Geometry: final body of the model. Coordinates: model frame, mm. Face numbers are marked on the shaded views. Round coordinates to 2 decimals unless told otherwise and drop trailing zeros. Order: outer loops, then holes, each group sorted by start corner. A loop starts at its lowest first (then second) coordinate and runs counter-clockwise, first axis right, second up. Notation, with made-up numbers: M 80,54.25 L 126,54.25 A19 cw 126,83.25 Z; hole C 89,18.25 d9. An arc over 180 degrees is marked long. Return JSON: item names as keys, results as strings. Group by question number.
Q1. Cut plane B-B on y = 15. Output: boundary loops of the cut face in (x, z).
Q2. Cut plane A-A on y = 10. Output: boundary loops of the cut face in (x, z), and give its area (3 significant figures).
Q3. Mould query, pull axis Y, two halves, no side actions, for the marked faces 1, 2 and 3. Classes: released by +Y, released by -Y, zero draft, split by the parting line, or undercut.
Q4. Ray query, probe 1 along X at (y, z) = (10, 2.15); probe 2 along X at (y, z) = (16, 2); probe 3 along Y at (x, z) = (14, 17.5) (3 decimals). Return the intervals inside material, ascending.
Q5. Contact query for flat-ended pins moving along their axis: pin 1 (2.5 mm diameter, centred on x = 15, y = 10, fed in from +Z); pin 2 (1.5 mm diameter, centred on x = 6, y = 11, fed in from -Z); pin 3 (10 mm diameter, centred on x = 8, y = 10.5, fed in from +Z); pin 4 (5.5 mm diameter, centred on y = 6.5, z = 1.5, fed in from -X). Output: stop coordinate, or through.
```python
from build123d import *

# Parameters (mm, degrees)
ESQUISSE1_W                                       = 10
ESQUISSE1_H                                       = 20
ESQUISSE1_W_2                                     = 20
BOSS_EXTRU_3_DEPTH                                = 5
BOSS_EXTRU_5_DEPTH                                = 2
ESQUISSE15_W                                      = 8
ESQUISSE15_H                                      = 17.913431031
BOSS_EXTRU_6_DEPTH                                = 0.1
ESQUISSE16_W                                      = 1
ESQUISSE16_H                                      = 17.913431031
BOSS_EXTRU_7_DEPTH                                = 1
BOSS_EXTRU_11_DEPTH                               = 2
ESQUISSE32_W                                      = 8
ESQUISSE32_H                                      = 17.913431031
BOSS_EXTRU_14_DEPTH                               = 0.125
ESQUISSE42_R                                      = 1.279103286
BOSS_EXTRU_18_DEPTH                               = 7
ESQUISSE56_R                                      = 1.3
BOSS_EXTRU_20_DEPTH                               = 7
CONG_4_R                                          = 1
ESQUISSE33_W                                      = 1
ESQUISSE33_H                                      = 17.913431031
BOSS_EXTRU_15_DEPTH                               = 1
ESQUISSE35_R                                      = 2.128247198
ENL_V_MAT_EXTRU_1_DEPTH                           = 5
ESQUISSE37_W                                      = 26
ESQUISSE37_H                                      = 16
ENL_V_MAT_EXTRU_2_DEPTH                           = 3
ESQUISSE38_R                                      = 3.5
BOSS_EXTRU_17_DEPTH                               = 3
ESQUISSE35_3_R                                    = 2.128247198
ENL_V_MAT_EXTRU_3_DEPTH                           = 5
FRAISAGE_POUR_VIS_T_TE_FRAIS_E_BOMB_E_D           = 3.7973
FRAISAGE_POUR_VIS_T_TE_FRAIS_E_BOMB_E_CSINK_D     = 7.0866
FRAISAGE_POUR_VIS_T_TE_FRAIS_E_BOMB_E_CSINK_ANGLE = 82


with BuildPart() as part:
    # Esquisse1 → Boss.-Extru.3 (new body)
    with BuildSketch(Plane.XY):
        with Locations((25, 10)):
            Rectangle(ESQUISSE1_W, ESQUISSE1_H)
        with Locations((10, 10)):
            Rectangle(ESQUISSE1_W_2, ESQUISSE1_H)
    extrude(amount=BOSS_EXTRU_3_DEPTH)

    # Esquisse14 → Boss.-Extru.5 (add)
    with BuildSketch(Plane(origin=(0, 20, 0), x_dir=(1, 0, 0), z_dir=(0, 1, 0))):
        Polygon((29.977520524, -4.978412673), (19.716916224, -33.169191296), (9.716916224, -33.169191296), (7.538022655, -8.264323844), (-0.022479476, -4.978412673), align=None)
    extrude(amount=-BOSS_EXTRU_5_DEPTH)

    # Esquisse15 → Boss.-Extru.6 (add)
    with BuildSketch(Plane(origin=(0, 18, 0), x_dir=(-1, 0, 0), z_dir=(0, -1, 0))):
        with Locations((-14.823599663, -13.956715516)):
            Rectangle(ESQUISSE15_W, ESQUISSE15_H)
    extrude(amount=BOSS_EXTRU_6_DEPTH)

    # Esquisse16 → Boss.-Extru.7 (add)
    with BuildSketch(Plane.XZ.offset(-17.9)):
        with Locations((12.323594191, 13.956715516)):
            Rectangle(ESQUISSE16_W, ESQUISSE16_H)
    extrude(amount=BOSS_EXTRU_7_DEPTH)



with BuildPart() as body_2:
    # Esquisse20 → Boss.-Extru.11 (new body)
    with BuildSketch(Plane(origin=(0, 0, 0), x_dir=(-1, 0, 0), z_dir=(0, -1, 0))):
        Polygon((0.007816785, -5.006477186), (-10.252787515, -33.19725581), (-20.252787515, -33.19725581), (-22.431681083, -8.292388358), (-29.992183215, -5.006477186), align=None)
    extrude(amount=-BOSS_EXTRU_11_DEPTH)


with BuildPart() as part_1:
    add(part.part)

    add(body_2.part)  # Boss.-Extru.14 merges body 2
    # Esquisse32 → Boss.-Extru.14 (add)
    with BuildSketch(Plane(origin=(0, 2, 0), x_dir=(1, 0, 0), z_dir=(0, 1, 0))):
        with Locations((14.516805055, -13.946251691)):
            Rectangle(ESQUISSE32_W, ESQUISSE32_H)
    extrude(amount=BOSS_EXTRU_14_DEPTH)

    # Esquisse42 → Boss.-Extru.18 (add)
    with BuildSketch(Plane(origin=(18.516805055, 0, 0), x_dir=(0, 0, -1), z_dir=(1, 0, 0))):
        with Locations((-30.710413968, 1.3)):
            Circle(ESQUISSE42_R)
    extrude(amount=-BOSS_EXTRU_18_DEPTH)

    # Esquisse56 → Boss.-Extru.20 (add)
    with BuildSketch(Plane(origin=(18.823599663, 0, 0), x_dir=(0, 0, -1), z_dir=(1, 0, 0))):
        with Locations((-30.475906609, 18.642606084)):
            Circle(ESQUISSE56_R)
    extrude(amount=-BOSS_EXTRU_20_DEPTH)

    # Congé4
    cong_4_edges = [part_1.edges().sort_by_distance(p)[0] for p in [
        (5.122485365, 2, 19.101866498),
        (5.122485365, 0, 19.101866498),
        (15.252787515, 0, 33.19725581),
        (15.252787515, 2, 33.19725581),
        (21.342234299, 2, 20.744822084),
        (21.342234299, 0, 20.744822084),
        (26.211932149, 2, 6.649432772),
        (26.211932149, 0, 6.649432772),
        (3.782606563, 18, 6.632161922),
        (3.782606563, 20, 6.632161922),
        (8.62746944, 18, 20.71675757),
        (8.62746944, 20, 20.71675757),
        (14.716916224, 18, 33.169191296),
        (14.716916224, 20, 33.169191296),
        (24.843289802, 18, 19.084595648),
        (24.843289802, 20, 19.084595648),
    ]]
    fillet(cong_4_edges, radius=CONG_4_R - 0.0001)  # a hair under: the kernel refuses the full size

    # Esquisse33 → Boss.-Extru.15 (add)
    with BuildSketch(Plane(origin=(0, 2.125, 0), x_dir=(-1, 0, 0), z_dir=(0, 1, 0))):
        with Locations((-12.203810405, 13.919189864)):
            Rectangle(ESQUISSE33_W, ESQUISSE33_H)
    extrude(amount=BOSS_EXTRU_15_DEPTH)

    # Esquisse35 → Enlèv. mat.-Extru.1 (cut)
    with BuildSketch(Plane.XY.offset(5)):
        with Locations((15, 10)):
            Circle(ESQUISSE35_R)
    extrude(amount=-ENL_V_MAT_EXTRU_1_DEPTH, mode=Mode.SUBTRACT)

    # Esquisse37 → Enlèv. mat.-Extru.2 (cut)
    with BuildSketch(Plane(origin=(0, 0, 0), x_dir=(-1, 0, 0), z_dir=(0, 0, -1))):
        with Locations((-15, 10)):
            Rectangle(ESQUISSE37_W, ESQUISSE37_H)
    extrude(amount=-ENL_V_MAT_EXTRU_2_DEPTH, mode=Mode.SUBTRACT)

    # Esquisse38 → Boss.-Extru.17 (add)
    with BuildSketch(Plane(origin=(0, 0, 3), x_dir=(-1, 0, 0), z_dir=(0, 0, -1))):
        with Locations(Location((-15, 10, 0), (0, 0, 180))):
            Circle(ESQUISSE38_R)
    extrude(amount=BOSS_EXTRU_17_DEPTH)

    # Esquisse35<3> → Enlèv. mat.-Extru.3 (cut)
    with BuildSketch(Plane.XY.offset(5)):
        with Locations((15, 10)):
            Circle(ESQUISSE35_3_R)
    extrude(amount=-ENL_V_MAT_EXTRU_3_DEPTH, mode=Mode.SUBTRACT)

    # Fraisage pour vis à tête fraisée bombée #61 (through all)
    with Locations(Plane.XY.offset(5)):
        with Locations((15, 10)):
            CounterSinkHole(FRAISAGE_POUR_VIS_T_TE_FRAIS_E_BOMB_E_D / 2, FRAISAGE_POUR_VIS_T_TE_FRAIS_E_BOMB_E_CSINK_D / 2, counter_sink_angle=FRAISAGE_POUR_VIS_T_TE_FRAIS_E_BOMB_E_CSINK_ANGLE)


solid = part_1.part
```
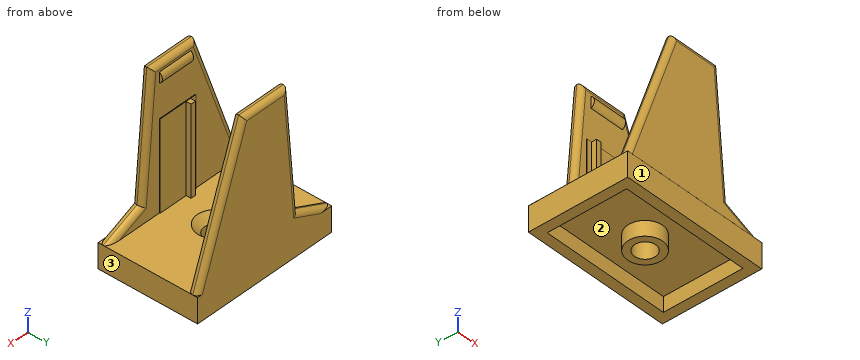
Result sheet:
{
 "1": {"outline": "M 0,0 L 2,0 L 2,3 L 28,3 L 28,0 L 30,0 L 30,5 L 0,5 Z"},
 "2": {"outline": "M 0,0 L 2,0 L 2,3 L 11.5,3 L 11.5,0 L 12.87,0 L 12.87,3.37 L 11.46,5 L 0,5 Z; M 17.13,0 L 18.5,0 L 18.5,3 L 28,3 L 28,0 L 30,0 L 30,5 L 18.54,5 L 17.13,3.37 Z", "area": "69.4 mm²"},
 "3": {"face 1": "released by -Y", "face 2": "undercut", "face 3": "zero draft"},
 "4": {"probe 1": "x = 0 to 2, 11.5 to 12.87, 17.13 to 18.5, 28 to 30", "probe 2": "x = 0 to 2, 28 to 30", "probe 3": "y = 0 to 2.125, 17.9 to 20"},
 "5": {"pin 1": "passes through", "pin 2": "stops at z = 3", "pin 3": "stops at z = 5", "pin 4": "stops at x = 0"}
}
